Design review of the part built by this model. Coordinates are the model's own, in mm. A direction names the side the tool comes from. Coordinates: 2 decimals unless noted, no trailing zeros. Loops run counter-clockwise (first coordinate to the right, second up) from the corner with the lowest first, then second, coordinate; pieces in that order, holes last. Notation, with made-up numbers: (57, 36.5) -> (75, 36.5) arc R18 cw to (75, 43.5) -> close; hole circle Ø11 at (-1.75, 24). An arc over 180 degrees is marked (long way). Answer in a Markdown table with one row per item.
```python
from build123d import *

# Parameters (mm, degrees)
F1_DEPTH = 15
F2_T     = -3
F3_R     = 5.08
F4_R     = 4
F5_DEPTH = 11.5
F6_R     = 1.95
F7_DEPTH = 10


with BuildPart() as f1:
    # F0 (on Top) → F1 (new body)
    with BuildSketch(Plane.XY):
        with BuildLine():
            ThreePointArc((-83.334517, -38.901611), (-81.474645, -43.391739), (-76.984517, -45.251611))
            Line((-76.984517, -45.251611), (75.315483, -45.251611))
            ThreePointArc((75.315483, -45.251611), (79.805611, -43.391739), (81.665483, -38.901611))
            Line((81.665483, -38.901611), (81.665483, 68.398389))
            ThreePointArc((81.665483, 68.398389), (79.805611, 72.888517), (75.315483, 74.748389))
            Line((75.315483, 74.748389), (-76.984517, 74.748389))
            ThreePointArc((-76.984517, 74.748389), (-81.474645, 72.888517), (-83.334517, 68.398389))
            Line((-83.334517, 68.398389), (-83.334517, -38.901611))
        make_face()
    extrude(amount=F1_DEPTH)

    # F2
    f2_openings = [f1.faces().sort_by_distance(p)[0] for p in [
        (-0.834517, 14.748389, 15),
    ]]
    offset(amount=F2_T, openings=f2_openings)

    # F3
    f3_edges = [f1.edges().sort_by_distance(p)[0] for p in [
        (-81.474645, 72.888517, 0),
    ]]
    fillet(f3_edges, radius=F3_R)

    # F4 (on face) → F5 (join)
    with BuildSketch(Plane.XY.offset(3)):
        with Locations((73.665483, -37.251611)):
            Circle(F4_R)
        with Locations((73.665483, 66.748389)):
            Circle(F4_R)
        with Locations((16.665483, 17.748389)):
            Circle(F4_R)
        with Locations((-75.334517, 39.748389)):
            Circle(F4_R)
        with Locations((-30.334517, -37.251611)):
            Circle(F4_R)
    extrude(amount=F5_DEPTH)

    # F6 (on face) → F7 (join)
    with BuildSketch(Plane.XY.offset(14.5)):
        with Locations((73.665483, -37.251611)):
            Circle(F6_R)
        with Locations((16.665483, 17.748389)):
            Circle(F6_R)
        with Locations((73.665483, 66.748389)):
            Circle(F6_R)
        with Locations((-30.334517, -37.251611)):
            Circle(F6_R)
        with Locations((-75.334517, 39.748389)):
            Circle(F6_R)
    extrude(amount=F7_DEPTH)


solid = f1.part
```
(1) Take a section at B-B on z = 22.25. Give the boundary of the cut face in (x, y).
Evaluation:
| item | result |
|---|---|
| outline | circle Ø3.9 at (-75.33, 39.75); circle Ø3.9 at (-30.33, -37.25); circle Ø3.9 at (16.67, 17.75); circle Ø3.9 at (73.67, -37.25); circle Ø3.9 at (73.67, 66.75) |
(2) Draft analysis for pull direction Y (two halves, no side actions). For faces 3 (the flat face through (-81, 15, 15)), 4 (the cylindrical face through (-1.9, 73.3, 1.53)), 5 (the flat face through (74, -35, 14.5)), 6 (the cylindrical face through (79.8, -43.4, 10)), state which applies: pulls with the +Y half, pulls with the -Y half, needs draft (parallel to the pull), parting line crosses it, or undercut.
Evaluation:
| item | result |
|---|---|
| face 3 | needs draft |
| face 4 | pulls with the +Y half |
| face 5 | undercut |
| face 6 | pulls with the -Y half |
(3) Take a section at A-A on z = 7.5. Give the boundary of the cut face in (x, y), and give its area (3 significant figures).
Evaluation:
| item | result |
|---|---|
| outline | (-83.33, -38.9) arc R6.35 ccw to (-76.98, -45.25) -> (75.32, -45.25) arc R6.35 ccw to (81.67, -38.9) -> (81.67, 68.4) arc R6.35 ccw to (75.32, 74.75) -> (-76.98, 74.75) arc R6.35 ccw to (-83.33, 68.4) -> close; circle Ø8 at (-75.33, 39.75); circle Ø8 at (-30.33, -37.25); circle Ø8 at (16.67, 17.75); circle Ø8 at (73.67, -37.25); circle Ø8 at (73.67, 66.75); hole (-80.33, -38.9) arc R3.35 ccw to (-76.98, -42.25) -> (75.32, -42.25) arc R3.35 ccw to (78.67, -38.9) -> (78.67, 68.4) arc R3.35 ccw to (75.32, 71.75) -> (-76.98, 71.75) arc R3.35 ccw to (-80.33, 68.4) -> close |
| area | 1,900 mm² |
(4) Take a section at D-D on y = 27.5. Give the boundary of the cut face in (x, z).
Evaluation:
| item | result |
|---|---|
| outline | (-83.33, 5.08) arc R5.08 ccw to (-78.25, 0) -> (76.59, 0) arc R5.08 ccw to (81.67, 5.08) -> (81.67, 15) -> (78.67, 15) -> (78.67, 3) -> (-80.33, 3) -> (-80.33, 15) -> (-83.33, 15) -> close |
(5) Take a section at C-C on x = -63.5. Give the boundary of the cut face in (y, z).
Evaluation:
| item | result |
|---|---|
| outline | (-45.25, 5.08) arc R5.08 ccw to (-40.17, 0) -> (69.67, 0) arc R5.08 ccw to (74.75, 5.08) -> (74.75, 15) -> (71.75, 15) -> (71.75, 3) -> (-42.25, 3) -> (-42.25, 15) -> (-45.25, 15) -> close |
(6) To check wall thickness, follow probe 1 along X at (y, z) = (46, 7.25); probe 2 along Y at (x, z) = (34.5, 6); probe 3 along Y at (x, z) = (-33.5, 7). State the ranges of each line that lie inside material, in increasing order.
Evaluation:
| item | result |
|---|---|
| probe 1 | x = -83.33 to -80.33, 78.67 to 81.67 |
| probe 2 | y = -45.25 to -42.25, 71.75 to 74.75 |
| probe 3 | y = -45.25 to -42.25, -39.7 to -34.81, 71.75 to 74.75 |
(7) Tool access review of faces 1 (the flat face through (17, 18, 24.5)), 2 (the cylindrical face through (-79.379, -41.244, 8.916)): name each direction out of +Z, -Z, +X, -X, +Y, -Y from which nothing blocks a thin tool from reaching the whole face with its end or side.
Evaluation:
| item | result |
|---|---|
| face 1 | +Z, +X, -X, +Y, -Y |
| face 2 | +Z |
(8) For pin 1 (8 mm diameter, centred on x = 16.5, y = 7.5, fed in from +Z); pin 2 (10 mm diameter, centred on x = -58.5, z = 21.5, fed in from +Y) (3 decimals), all flat-tipped, find the tip position at first contact; note any pin that passes through.
Evaluation:
| item | result |
|---|---|
| pin 1 | stops at z = 3 |
| pin 2 | passes through |
